Autodesk Inventor part; units mm, degrees
ref_plane "Work Plane1" through (3.7, 0, 0) normal (0, 0, 1) x (1, 0, 0)
ref_plane "YZ Plane" through (0, 0, 0) normal (1, 0, 0) x (0, 1, 0)
ref_plane "XZ Plane" through (0, 0, 0) normal (0, 1, 0) x (-1, 0, 0)
sketch "Sketch1" plane through (0, 0, 0) normal (0, 1, 0) x (-1, 0, 0)
  line L0 (0, 0) -> (-3.7, 0)
  line L1 (-3.7, 0) -> (-5.7, 0)
  line L2 (0, 0) -> (0, -40.75)
  line L3 (0, -40.75) -> (0, -50.75)
  circle A0 centre (0, -50.75) radius 10
  line L4 (-1.5, -40.8631) -> (0, -40.8631)
  line L5 (0, -40.8631) -> (0, -40.75)
  line L6 (-1.5, -40.75) -> (-1.5, -40.8631)
  line L7 (-1.5, -40.8631) -> (-3.7, 0)
  line L8 (0, -40.75) -> (-1.5, -40.75)
  line L9 (-1.5, -40.75) -> (-2, -40.75)
  line L10 (-2, -40.75) -> (-2, -40.952)
  line L11 (-2, -40.952) -> (-5.7, 0)
  line L12 (0, -50.75) -> (0, -60.75)
  circle A1 centre (0, -50.75) radius 9.2
  line L13 (-1.5, -40.8631) -> (-1.4568, -41.6661)
  line L14 (-3.7, 0) -> (-3.7, 15)
  line L15 (-3.7, 15) -> (-0.2, 15)
  line L16 (-5.7, 0) -> (-5.7, 15)
  line L17 (-5.7, 15) -> (-3.7, 15)
  point P0 (0, -59.95)
  dimension "d7" = 18.4
  dimension "d0" = 3.7
  dimension "d1" = 2
  dimension "d2" = 40.75
  dimension "d4" = 10
  dimension "d6" = 0.5
  dimension "d9" = 15
revolve "Revolution1" add sketch "Sketch1" angle 180 about axis through (0, 0, 0) along (0, 0, 1) contours L7 L9 L10 L11 L1 | L1 L16 L17 L14 | L7 A0 L10 L9 | L13 A1 L12 A0
ref_plane "Work Plane1" through (3.7, 0, 0) normal (0, 0, 1) x (1, 0, 0)
sketch "Sketch2" plane through (3.7, 0, 0) normal (0, 0, 1) x (1, 0, 0)
  circle A0 centre (-3.7, 0) radius 3.7
  circle A1 centre (-3.7, 0) radius 2.2
  line L0 (2, 0) -> (-1.7, 0)
  line L1 (0, 0) -> (-7.4, 0)
  point P0 (-5.9, 0)
  point P1 (-1.5, 0)
  dimension "d13" = 4.4
  dimension "d14" = 7.4
extrude "Rod Stopper" add sketch "Sketch2" against normal blind 2 contours L0 A1 L1 A0 picked at (-6.8429, 0.4707)
fillet "Fillet1" radius 2 1 edges at (0, 2, -40.952)
properties part number "markerWithRodEnd_3DPrint"
The model under review builds one solid part; all positions refer to its coordinate system, in mm. A direction names the side the tool comes from. Round coordinates to 2 decimals unless told otherwise and drop trailing zeros. Write each loop counter-clockwise with the first axis right and the second up, starting at its lowest first coordinate (ties: lowest second). Pieces come first, ordered by that corner, then holes. Notation, with made-up numbers: (15.25, 66.5) - (36.25, 66.5) arc R20 cw to (36.25, 76.5) - close; hole circle Ø6 at (49, 7.25). An arc over 180 degrees is marked (long way). One line per question, with ' | ' between items.
Item 1: Add section A-A, the plane z = 5. Give the boundary of the cut face in (x, y).
Resolved:
outline: (-5.7, 0) - (-3.7, 0) arc R3.7 cw to (3.7, 0) - (5.7, 0) arc R5.7 ccw to start
Item 2: Add section C-C, the plane x = 7. Give the boundary of the cut face in (y, z).
Resolved:
outline: (0, -57.89) arc R7.14 ccw to (0, -43.61) - (0, -44.78) arc R5.97 cw to (0, -56.72) - close
Item 3: To check wall thickness, follow probe 1 along Z at (x, y) = (6.5, 1); probe 2 along X at (y, z) = (7.25, -53); probe 3 along X at (y, z) = (6.75, -56). State the ranges of each line that lie inside material, in increasing order.
Resolved:
probe 1: z = -58.28 to -57.18, -44.32 to -43.22 | probe 2: x = -6.51 to -5.2, 5.2 to 6.51 | probe 3: x = -5.18 to -3.39, 3.39 to 5.18
Item 4: Add section B-B, the plane y = 7.25. Give the boundary of the cut face in (x, z).
Resolved:
outline: circle Ø13.77 at (0, -50.75); hole circle Ø11.33 at (0, -50.75)
Item 5: For P1, Ø1.1, axis at x = 0.5, y = 1, coming from the -Z side; P2, Ø2, axis at x = -1.5, z = -6.5, coming from the +Y side; P3, Ø1.5, axis at x = -7.5, y = 2, coming from the +Z side; P4, Ø1.5, axis at x = -4.5, z = -24.5, coming from the -Y side, all flat-tipped, find the tip position at first contact; note any pin that passes through.
Resolved:
P1: stops at z = -60.73 | P2: stops at y = 5.12 | P3: stops at z = -43.62 | P4: passes through
Item 6: The part is to be moulded in two halves that separate along Z. For faces 4 (the face through (0.1, 5.7, 7.6)), 5 (the face through (0, 3, -2)), 6 (the face through (0, 3, 0)), say which applies: pulls with the +Z half, pulls with the -Z half, needs draft (parallel to the pull), parting line crosses it, or undercut.
Resolved:
face 4: needs draft | face 5: undercut | face 6: pulls with the +Z half
Item 7: For faces 1 (the face through (0, 2.2, -1)), 2 (the face through (3, 0, -17)), 3 (the face through (0.09, 3.95, -19.38)), list the 3-axis set-ups (+Z, -Z, +X, -X, +Y, -Y) from which the entire face can be reached by the end or side of a thin tool; tool diameter is ignored.
Resolved:
face 1: +Z, -Y | face 2: +Z, -Z, +X, -X, -Y | face 3: +Y
